from build123d import *

# Parameters (mm, degrees)
MODEL_R                 = 1.7
MODEL_R_2               = 1.600279216
SALIENTE_EXTRUIR1_DEPTH = 3


with BuildPart() as part:
    # Model → Saliente-Extruir1 (new body)
    with BuildSketch(Plane.XY):
        with BuildLine():
            Line((74.679802956, 300.758040435), (5.677398721, 300.758040435))
            ThreePointArc((5.677398721, 300.758040435), (4.61673855, 300.318700606), (4.177398721, 299.258040435))
            Line((4.177398721, 299.258040435), (4.177398721, 221.253430577))
            ThreePointArc((4.177398721, 221.253430577), (4.61673855, 220.192770405), (5.677398721, 219.753430577))
            Line((5.677398721, 219.753430577), (74.679802956, 219.753430577))
            ThreePointArc((74.679802956, 219.753430577), (75.740463127, 220.192770405), (76.179802956, 221.253430577))
            Line((76.179802956, 221.253430577), (76.179802956, 299.258040435))
            ThreePointArc((76.179802956, 299.258040435), (75.740463127, 300.318700606), (74.679802956, 300.758040435))
        make_face()
        with Locations((17.676729717, 224.253096075)):
            Circle(MODEL_R, mode=Mode.SUBTRACT)
        with Locations((62.680137458, 224.253096075)):
            Circle(MODEL_R, mode=Mode.SUBTRACT)
        with Locations((8.677064219, 224.253096075)):
            Circle(MODEL_R_2, mode=Mode.SUBTRACT)
        with Locations((71.679802956, 224.253096075)):
            Circle(MODEL_R_2, mode=Mode.SUBTRACT)
        with Locations((17.676729717, 296.258040435)):
            Circle(MODEL_R, mode=Mode.SUBTRACT)
        with Locations((62.680137458, 296.258040435)):
            Circle(MODEL_R, mode=Mode.SUBTRACT)
        with Locations((71.679802956, 296.258040435)):
            Circle(MODEL_R_2, mode=Mode.SUBTRACT)
        with Locations((8.677064219, 296.258040435)):
            Circle(MODEL_R_2, mode=Mode.SUBTRACT)
        with BuildLine():
            Line((73.679621744, 292.260238845), (73.679621744, 227.755628988))
            ThreePointArc((73.679621744, 227.755628988), (73.386728525, 227.048522207), (72.679621744, 226.755628988))
            Line((72.679621744, 226.755628988), (60.179621744, 226.755628988))
            ThreePointArc((60.179621744, 226.755628988), (59.472514963, 226.462735769), (59.179621744, 225.755628988))
            Line((59.179621744, 225.755628988), (59.179621744, 225.165628988))
            ThreePointArc((59.179621744, 225.165628988), (58.886728525, 224.458522207), (58.179621744, 224.165628988))
            Line((58.179621744, 224.165628988), (30.17721751, 224.165628988))
            ThreePointArc((30.17721751, 224.165628988), (29.470110728, 224.458522207), (29.17721751, 225.165628988))
            Line((29.17721751, 225.165628988), (29.17721751, 227.730037779))
            ThreePointArc((29.17721751, 227.730037779), (28.884324291, 228.43714456), (28.17721751, 228.730037779))
            Line((28.17721751, 228.730037779), (7.67721751, 228.730037779))
            ThreePointArc((7.67721751, 228.730037779), (6.970110728, 229.022930998), (6.67721751, 229.730037779))
            Line((6.67721751, 229.730037779), (6.67721751, 291.370238846))
            ThreePointArc((6.67721751, 291.370238846), (6.970110728, 292.077345627), (7.67721751, 292.370238846))
            Line((7.67721751, 292.370238846), (19.67721751, 292.370238846))
            ThreePointArc((19.67721751, 292.370238846), (20.384324291, 292.663132064), (20.67721751, 293.370238846))
            Line((20.67721751, 293.370238846), (20.67721751, 297.097066693))
            ThreePointArc((20.67721751, 297.097066693), (20.970110728, 297.804173474), (21.67721751, 298.097066693))
            Line((21.67721751, 298.097066693), (58.179621744, 298.097066693))
            ThreePointArc((58.179621744, 298.097066693), (58.886728525, 297.804173474), (59.179621744, 297.097066693))
            Line((59.179621744, 297.097066693), (59.179621744, 294.260238845))
            ThreePointArc((59.179621744, 294.260238845), (59.472514963, 293.553132064), (60.179621744, 293.260238845))
            Line((60.179621744, 293.260238845), (72.679621744, 293.260238845))
            ThreePointArc((72.679621744, 293.260238845), (73.386728525, 292.967345627), (73.679621744, 292.260238845))
        make_face(mode=Mode.SUBTRACT)
    extrude(amount=SALIENTE_EXTRUIR1_DEPTH)


solid = part.part
Verification items for the finished model (mm, model axes). A direction names the side the tool comes from. Give positions to 0.01 mm unless a question says otherwise; leave off trailing zeros. Write each loop counter-clockwise with the first axis right and the second up, starting at its lowest first coordinate (ties: lowest second). Pieces come first, ordered by that corner, then holes. Notation, with made-up numbers: M 23,45 L 56,45 A16 ccw 56,51 Z; hole C -1,7 d5. An arc over 180 degrees is marked long. Write item = value, one per line.
(1) Sectioned sample at B-B (y = 288). Record the cut outline in (x, z), then the cut area to 3 significant figures.
Found:
outline = M 4.18,0 L 6.68,0 L 6.68,3 L 4.18,3 Z; M 73.68,0 L 76.18,0 L 76.18,3 L 73.68,3 Z
area = 15.0 mm2
(2) Sectioned sample at A-A (x = 13). Record the cut outline in (y, z), then the cut area to 3 significant figures.
Found:
outline = M 219.75,0 L 228.73,0 L 228.73,3 L 219.75,3 Z; M 292.37,0 L 300.76,0 L 300.76,3 L 292.37,3 Z
area = 52.1 mm2
(3) Sectioned sample at C-C (z = 0.8). Give the number of separate pieces and of enclosed holes in the cut face, then the cut area to 3 significant figures.
Found:
separate_pieces = 1
enclosed_holes = 9
area = 1,100 mm2
(4) Access from +Z, -Z, +X, -X, +Y, -Y to the whole of each face (thin tool, end or side, straight path). Record for faces 1 (the face through (29.177, 226, 1)), 2 (the face through (41, 300.758, 1)).
Found:
face_1 = +Z, -Z
face_2 = +Z, -Z, +X, -X, +Y
(5) Material ranges on line 1 (X direction, y = 296, z = 2.6); line 2 (Y direction, x = 35, z = 2.2); line 3 (X direction, y = 297, z = 1.9), recorded low to high.
Found:
line_1 = 4.18 to 7.1, 10.26 to 16, 19.36 to 20.68, 59.18 to 61, 64.36 to 70.1, 73.26 to 76.18
line_2 = 219.75 to 224.17, 298.1 to 300.76
line_3 = 4.18 to 7.26, 10.09 to 16.15, 19.21 to 20.68, 59.18 to 61.15, 64.21 to 70.26, 73.1 to 76.18
(6) Draft check along Y on faces 3 (the face through (14, 292.37, 1)), 4 (the face through (76.18, 260, 1)), 5 (the face through (40, 219.753, 1)). Enter one of: released by +Y, released by -Y, zero draft, split by the parting line, or undercut.
Found:
face_3 = undercut
face_4 = zero draft
face_5 = released by -Y
